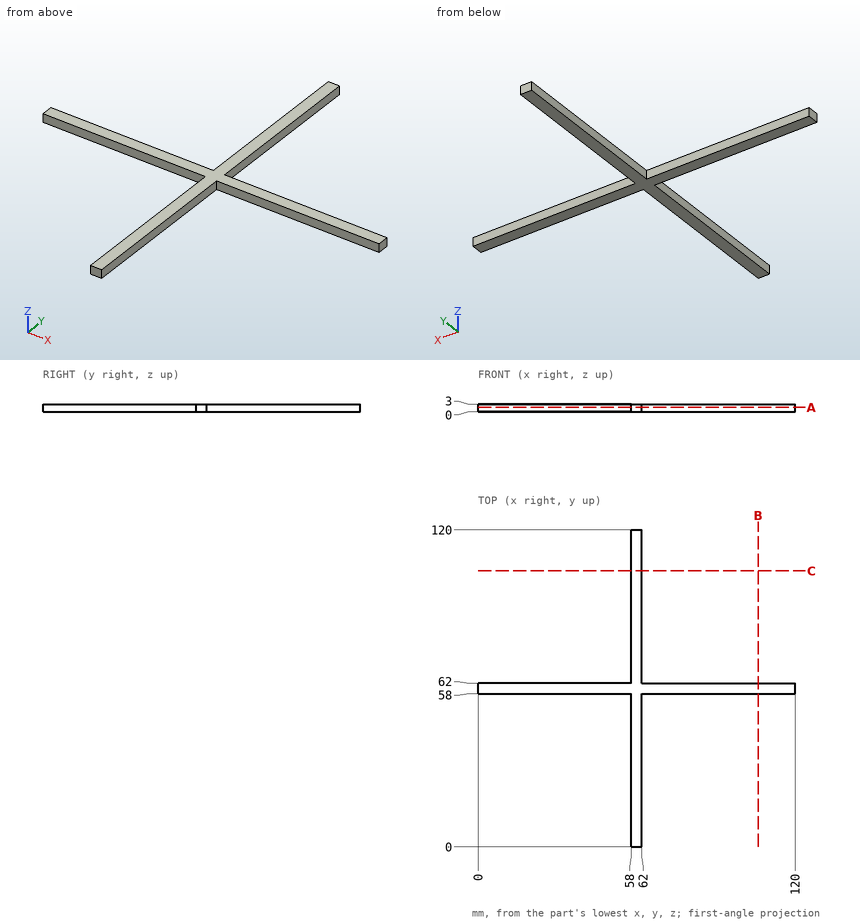
Study the drawing (mm; zero at the part's minimum x, y, z) and answer. Round coordinates to 2 decimals unless told otherwise and drop trailing zeros. Write each loop counter-clockwise with the first axis right and the second up, starting at its lowest first coordinate (ties: lowest second). Pieces come first, ordered by that corner, then holes. Notation, with made-up numbers: (28, -13) -> (32, -13) arc R28 ccw to (32, 17) -> close; hole circle Ø4 at (-32, -26). An arc over 180 degrees is marked (long way). Write item = value, one per line.
1) A straight line is drawn through the part: line 1 along Y through (x, z) = (66, 0.9). Find the intervals that lie inside material, in ascending order. Write a range as [from, to].
Check values:
line_1 = [58, 62]
2) Section A-A on z = 1.75 is taken. Write down the section's boundary in (x, y).
Check values:
outline = (0, 58) -> (58, 58) -> (58, 0) -> (62, 0) -> (62, 58) -> (120, 58) -> (120, 62) -> (62, 62) -> (62, 120) -> (58, 120) -> (58, 62) -> (0, 62) -> close
3) Given pin 1 (1.5 mm diameter, centred on y = 18, z = 1, fed in from -X); pin 2 (0.9 mm diameter, centred on x = 99.5, z = 1, fed in from -Y); pin 3 (0.9 mm diameter, centred on x = 100.5, z = 1.5, fed in from +Y); pin 4 (2 mm diameter, centred on x = 63.5, y = 104.5, fed in from +Z), each flat-ended and moving along its own axis, determine where each tip first touches the part or whether it passes through.
Check values:
pin_1 = 58
pin_2 = 58
pin_3 = 62
pin_4 = through
4) Section B-B on x = 106 is taken. Write down the section's boundary in (y, z).
Check values:
outline = (58, 0) -> (62, 0) -> (62, 3) -> (58, 3) -> close
